from build123d import *

# Parameters (mm, degrees)
SALIENTE_EXTRUIR1_DEPTH        = 3
REDONDEO1_R                    = 30
CORTAR_EXTRUIR1_DEPTH          = 156.335310697
TALADRO_DE_MARGEN_PARA_M31_D   = 3.4
CROQUIS16_W                    = 50.8
CROQUIS16_H                    = 33
CORTAR_EXTRUIR2_DEPTH          = 156.335310697
TALADRO_DE_MARGEN_PARA_M3_51_D = 3.9


with BuildPart() as part:
    # Croquis1 → Saliente-Extruir1 (new body)
    with BuildSketch(Plane.XY):
        Polygon((72.862780289, -137.153468779), (-72.862780289, -137.153468779), (-72.862780289, -77.415075694), (-43.862780289, -37.5), (-43.862780289, 37.5), (-72.862780289, 77.415075694), (-72.862780289, 137.153468779), (72.862780289, 137.153468779), (72.862780289, 77.415075694), (43.862780289, 37.5), (43.862780289, -37.5), (72.862780289, -77.415075694), align=None)
    extrude(amount=SALIENTE_EXTRUIR1_DEPTH)

    # Redondeo1
    redondeo1_edges = [part.edges().sort_by_distance(p)[0] for p in [
        (72.862780289, 77.415075694, 1.5),
        (43.862780289, 37.5, 1.5),
        (43.862780289, -37.5, 1.5),
        (72.862780289, -77.415075694, 1.5),
        (-72.862780289, -77.415075694, 1.5),
        (-43.862780289, -37.5, 1.5),
        (-43.862780289, 37.5, 1.5),
        (-72.862780289, 77.415075694, 1.5),
    ]]
    fillet(redondeo1_edges, radius=REDONDEO1_R)

    # Croquis2 → Cortar-Extruir1 (cut, through all)
    with BuildSketch(Plane.XY.offset(3)):
        with BuildLine():
            Line((-7.5, 45), (-7.5, 65))
            ThreePointArc((-7.5, 65), (0, 72.5), (7.5, 65))
            Line((7.5, 65), (7.5, 45))
            ThreePointArc((7.5, 45), (0, 37.5), (-7.5, 45))
        make_face()
    cortar_extruir1 = extrude(amount=-CORTAR_EXTRUIR1_DEPTH, mode=Mode.SUBTRACT)

    # Simetría1: Cortar-Extruir1 across plane
    add(cortar_extruir1.mirror(Plane.ZX), mode=Mode.SUBTRACT)

    # Taladro de margen para M31 (through all)
    with Locations(Plane.XY.offset(3)):
        with Locations((-56.662780289, 127.153468779), (-18.162780289, 127.153468779), (-18.162780289, 87.153468779), (-56.662780289, 87.153468779), (20.462780289, 127.153468779), (20.462780289, 87.153468779), (58.962780289, 87.153468779), (58.962780289, 127.153468779), (58.962780289, -123.153468779), (20.462780289, -123.153468779), (20.462780289, -83.153468779), (58.962780289, -83.153468779), (-18.162780289, -123.153468779), (-56.662780289, -123.153468779), (-56.662780289, -83.153468779), (-18.162780289, -83.153468779)):
            Hole(TALADRO_DE_MARGEN_PARA_M31_D / 2)

    # Croquis16 → Cortar-Extruir2 (cut, through all)
    with BuildSketch(Plane(origin=(0, 0, 0), x_dir=(-1, 0, 0), z_dir=(0, 0, -1))):
        with Locations((-38.562780289, 107.903468779)):
            Rectangle(CROQUIS16_W, CROQUIS16_H)
        with Locations((38.562780289, 107.903468779)):
            Rectangle(CROQUIS16_W, CROQUIS16_H)
        with Locations((38.562780289, -102.403468779)):
            Rectangle(CROQUIS16_W, CROQUIS16_H)
        with Locations((-38.562780289, -102.403468779)):
            Rectangle(CROQUIS16_W, CROQUIS16_H)
    extrude(amount=-CORTAR_EXTRUIR2_DEPTH, mode=Mode.SUBTRACT)

    # Taladro de margen para M3.51 (through all)
    with Locations(Plane.XY.offset(3)):
        with Locations((-58, 71), (0, 110), (-58, -71), (0, -130), (58, -71), (58, 71)):
            Hole(TALADRO_DE_MARGEN_PARA_M3_51_D / 2)


solid = part.part
The model under review builds one solid part; all positions refer to its coordinate system, in mm. A direction names the side the tool comes from. Give positions to 0.01 mm unless a question says otherwise; leave off trailing zeros. Order: outer loops, then holes, each group sorted by start corner. A loop starts at its lowest first (then second) coordinate and runs counter-clockwise, first axis right, second up. Notation, with made-up numbers: (70.5, 34.5) -> (78.5, 34.5) arc R22 ccw to (78.5, 68.5) -> close; hole circle Ø11 at (-35.75, 40.25). An arc over 180 degrees is marked (long way). Write item = value, one per line. Start each with the question number.
(1) Take a section at B-B (y = 52). Write out the cut boundary in (x, z), plus the area to 3 significant figures.
(2) Take a section at D-D (z = 2.25). State how many separate pieces and enclosed holes the cut face has, plus the area to 3 significant figures.
(3) Draft analysis for pull direction X (two halves, no side actions). For faces 5 (the cylindrical face through (-0.16, -72.5, 1.52)), 6 (the cylindrical face through (-45.372, -37.148, 1.521)), 7 (the flat face through (58.49, 57.63, 1.48)), 8 (the cylindrical face through (-0.16, 72.5, 1.52)), state which applies: +X half, -X half, draft (parallel to the pull), parting line (faces both ways), or undercut.
(4) For pin 1 Ø4 at (x, y) = (-56.66, -123.15) entering from -Z, flat-tipped, find the tip position at first contact; note if it passes through.
(5) Take a section at C-C (y = -24). Write out the cut boundary in (x, z), plus the area to 3 significant figures.
(6) Take a section at A-A (x = -38). Write out the cut boundary in (y, z).
(7) For L1, parallel to Y at x = 32.5, z = 0.6; L2, parallel to X at y = -93, z = 0.2; L3, parallel to Y at x = 57, z = 2.35, list the stretches that pass through material, from the lowest coordinate up. Write a range as from..to.
(8) Tool access review of faces 1 (the flat face through (58.24, -57.29, 1.48)), 2 (the cylindrical face through (-71.435, -78.018, 1.521)), 3 (the cylindrical face through (0.16, -37.5, 1.52)), 4 (the flat face through (1, -29, 0)): name each direction out of +Z, -Z, +X, -X, +Y, -Y from which nothing blocks a thin tool from reaching the whole face with its end or side.
Returned:
q1.outline = (-54.4, 0) -> (-7.5, 0) -> (-7.5, 3) -> (-54.4, 3) -> close; (7.5, 0) -> (54.4, 0) -> (54.4, 3) -> (7.5, 3) -> close
q1.area = 281 mm²
q2.separate_pieces = 1
q2.enclosed_holes = 28
q2.area = 25,400 mm²
q3.face_5 = undercut
q3.face_6 = -X half
q3.face_7 = +X half
q3.face_8 = undercut
q4.pin_1 = 0
q5.outline = (-43.86, 0) -> (43.86, 0) -> (43.86, 3) -> (-43.86, 3) -> close
q5.area = 263 mm²
q6.outline = (-137.15, 0) -> (-118.9, 0) -> (-118.9, 3) -> (-137.15, 3) -> close; (-85.9, 0) -> (91.4, 0) -> (91.4, 3) -> (-85.9, 3) -> close; (124.4, 0) -> (137.15, 0) -> (137.15, 3) -> (124.4, 3) -> close
q7.L1 = -137.15..-118.9, -85.9..91.4, 124.4..137.15
q7.L2 = -72.86..-63.96, -13.16..13.16, 63.96..72.86
q7.L3 = -137.15..-118.9, -85.9..-72.67, -69.33..-55.58, 55.58..69.33, 72.67..91.4, 124.4..137.15
q8.face_1 = +Z, -Z, +X
q8.face_2 = +Z, -Z, -X
q8.face_3 = +Z, -Z
q8.face_4 = -Z, +X, -X, +Y, -Y
